Drawing for the job (mm, zero at the part's lowest x, y, z). Round coordinates to 2 decimals unless told otherwise and drop trailing zeros. Order: outer loops, then holes, each group sorted by start corner. A loop starts at its lowest first (then second) coordinate and runs counter-clockwise, first axis right, second up. Notation, with made-up numbers: (51.25, 73) -> (77.25, 73) arc R10 ccw to (77.25, 87) -> close; hole circle Ø1 at (72.25, 12). An arc over 180 degrees is marked (long way). Use CSV: the item, a comma, the result in double quotes.
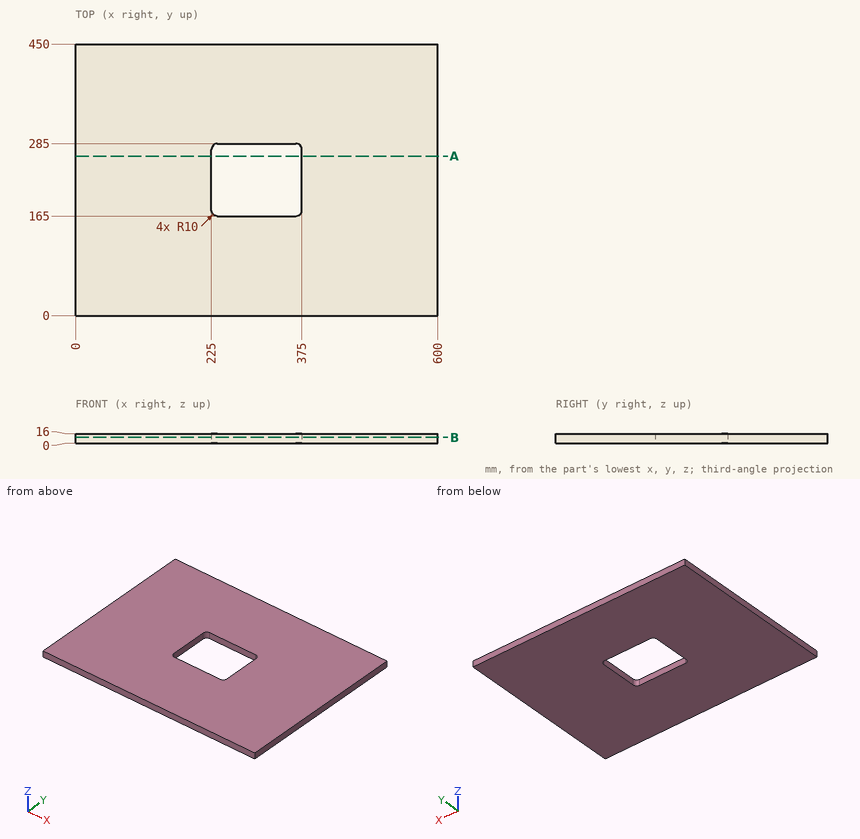
Q1. Pin check, flat tip, straight feed: pin 1 (1.5 mm diameter, centred on x = 113.5, y = 353, fed in from -Z). Stop position of the tip, or through.
From the geometry:
pin 1,"stops at z = 0"
Q2. Cut at B-B (z = 9.75). Give the cut face in (x, y), plus the area to 3 significant figures.
From the geometry:
outline,"(0, 0) -> (600, 0) -> (600, 450) -> (0, 450) -> close; hole (225, 175) arc R10 ccw to (235, 165) -> (365, 165) arc R10 ccw to (375, 175) -> (375, 275) arc R10 ccw to (365, 285) -> (235, 285) arc R10 ccw to (225, 275) -> close"
area,"252,000 mm²"
Q3. Cut at A-A (y = 264.5). Give the cut face in (x, z), plus the area to 3 significant figures.
From the geometry:
outline,"(0, 0) -> (225, 0) -> (225, 16) -> (0, 16) -> close; (375, 0) -> (600, 0) -> (600, 16) -> (375, 16) -> close"
area,"7,200 mm²"
Q4. Probe line 1 along X through (y, z) = (273, 1.25); line 2 along Y through (x, z) = (284, 4.75); line 3 along Y through (x, z) = (369, 4.25). List the from-to ranges inside material, lowest first.
From the geometry:
line 1,"x = 0 to 225, 375 to 600"
line 2,"y = 0 to 165, 285 to 450"
line 3,"y = 0 to 165.83, 284.17 to 450"
